Autodesk Inventor part; units mm, degrees
ref_plane "YZ Plane" through (0, 0, 0) normal (1, 0, 0) x (0, 1, 0)
ref_plane "XZ Plane" through (0, 0, 0) normal (0, 1, 0) x (-1, 0, 0)
ref_plane "XY Plane" through (0, 0, 0) normal (0, 0, 1) x (1, 0, 0)
sketch "スケッチ1" plane through (0, 0, 0) normal (0, 1, 0) x (-1, 0, 0)
  circle A0 centre (0, 0) radius 178.1675
  circle A1 centre (0, 0) radius 157.8276
  line L0 (168.1877, 0) -> (166.7488, -21.9529)
  line L1 (168.1877, 0) -> (130.1721, 2.4917) construction
  line L2 (249.4344, 0) -> (-249.4344, 0)
  line L3 (166.7488, -21.9529) -> (156.7702, -21.2989)
  line L4 (156.7702, -21.2989) -> (158.2091, 0.654) construction
  line L5 (158.2091, 0.654) -> (168.1877, 0)
  line L6 (157.4896, -10.3224) -> (0, 0)
  line L7 (166.7488, -21.9529) -> (162.4568, -43.5302)
  line L8 (162.4568, -43.5302) -> (152.649, -41.5793) construction
  line L9 (152.649, -41.5793) -> (156.9409, -20.002) construction
  line L10 (156.9409, -20.002) -> (166.7488, -21.9529) construction
  line L11 (162.4568, -43.5302) -> (155.3851, -64.3626)
  line L12 (155.3851, -64.3626) -> (145.9158, -61.1482) construction
  line L13 (145.9158, -61.1482) -> (152.9875, -40.3158) construction
  line L14 (152.9875, -40.3158) -> (162.4568, -43.5302) construction
  line L15 (155.3851, -64.3626) -> (145.6548, -84.0938)
  line L16 (145.6548, -84.0938) -> (136.6861, -79.6709) construction
  line L17 (136.6861, -79.6709) -> (146.4164, -59.9397) construction
  line L18 (146.4164, -59.9397) -> (155.3851, -64.3626) construction
  line L19 (0, 0) -> (111.6009, -111.6009)
  line L20 (145.6548, -84.0938) -> (137.3401, -78.5381) construction
  line L21 (137.3401, -78.5381) -> (125.1176, -96.8305) construction
  line L22 (125.1176, -96.8305) -> (133.4323, -102.3862) construction
  line L23 (133.4323, -102.3862) -> (145.6548, -84.0938)
  line L24 (133.4323, -102.3862) -> (125.9139, -95.7927) construction
  line L25 (125.9139, -95.7927) -> (111.4082, -112.3332) construction
  line L26 (111.4082, -112.3332) -> (118.9266, -118.9266)
  line L27 (118.9266, -118.9266) -> (133.4323, -102.3862)
  line L28 (111.6009, -111.6009) -> (118.9266, -118.9266)
  line L29 (166.7488, -21.9529) -> (176.7274, -22.6069) construction
  line L30 (118.9266, -118.9266) -> (125.9834, -125.9834)
  point P0 (154.795, -30.7906)
  point P1 (149.4517, -50.732)
  point P2 (141.5512, -69.8053)
  point P3 (131.2288, -87.6843)
  point P4 (118.661, -104.0629)
  point P5 (157.8276, 0)
  point P6 (178.1675, 0)
  dimension "d0" = 22
  dimension "d1" = 10
  dimension "d2" = 45
  dimension "d4" = 315.6551
extrude "押し出し1" add sketch "スケッチ1" along normal blind 5.5 contours L30 L27 L23 L15 L11 L7 L0 L2 A0 | L28 A1 L2 L0 L7 L11 L15 L23 L27
sketch "スケッチ2" plane through (0, 5.5, 0) normal (0, 1, 0) x (1, 0, 0)
  circle A0 centre (0, 0) radius 277.8276
  line L0 (-168.1877, 0) -> (-166.7488, 21.9529)
  line L1 (-166.7488, 21.9529) -> (-162.4568, 43.5302)
  line L2 (-162.4568, 43.5302) -> (-155.3851, 64.3626)
  line L3 (-155.3851, 64.3626) -> (-145.6548, 84.0938)
  line L4 (-133.4323, 102.3862) -> (-145.6548, 84.0938)
  line L5 (-118.9266, 118.9266) -> (-133.4323, 102.3862)
  line L6 (-167.4682, 10.9764) -> (-166.0294, 32.9293)
  line L7 (-166.0294, 32.9293) -> (-275.7938, 40.1237)
  line L8 (-275.7938, 40.1237) -> (-277.2327, 18.1708)
  line L9 (-277.2327, 18.1708) -> (-167.4682, 10.9764)
  line L10 (-164.6028, 32.7415) -> (-160.3108, 54.3188)
  line L11 (-160.3108, 54.3188) -> (-268.1972, 75.7787)
  line L12 (-268.1972, 75.7787) -> (-272.4892, 54.2015)
  line L13 (-272.4892, 54.2015) -> (-164.6028, 32.7415)
  circle A1 centre (-166.7488, 21.9529) radius 11
  circle A2 centre (-162.4568, 43.5302) radius 11
  line L14 (-158.921, 53.9464) -> (-151.8493, 74.7789)
  line L15 (-151.8493, 74.7789) -> (-256.0116, 110.1372)
  line L16 (-256.0116, 110.1372) -> (-263.0833, 89.3047)
  line L17 (-263.0833, 89.3047) -> (-158.921, 53.9464)
  circle A3 centre (-155.3851, 64.3626) radius 11
  arc A4 (-275.7591, 62.4834) -> (-281.3553, 41.7349) centre (-166.7488, 21.9529) ccw
  line L18 (-178.1663, 0.654) -> (-158.2091, -0.654)
  line L19 (-158.2091, -0.654) -> (-156.7702, 21.2989)
  line L20 (-156.7702, 21.2989) -> (-176.7274, 22.6069)
  line L21 (-176.7274, 22.6069) -> (-178.1663, 0.654)
  line L22 (-177.4468, 11.6305) -> (-275.7938, 40.1237)
  line L23 (-176.7274, 22.6069) -> (-176.008, 33.5834)
  line L24 (-176.008, 33.5834) -> (-275.7591, 62.4834)
  line L25 (-275.7938, 40.1237) -> (-281.3553, 41.7349)
  circle A5 centre (0, 0) radius 137.8276
  line L26 (0, 0) -> (-196.4538, 196.4538)
  line L27 (-111.6009, 111.6009) -> (-125.9834, 125.9834)
  line L28 (-433.7586, 0) -> (433.7586, 0)
  circle A6 centre (0, 0) radius 257.8276 construction
  arc A7 (-111.6009, 111.6009) -> (-157.8276, 0) centre (0, 0) ccw
  point P0 (-158.1662, 0)
  point P1 (-137.8276, 0)
  point P2 (-97.4588, 97.4588)
  point P3 (-277.8276, 0)
  dimension "d7" = 22
  dimension "d10" = 20
  dimension "d11" = 100
  dimension "d12" = 20
  dimension "d14" = 20
  dimension "d17" = 100
extrude "押し出し2" add sketch "スケッチ2" against normal blind 5.5 contours L26 L5 L4 L3 A3 L15 A0 | A0 L9 L21 L18 L28 | L15 A3 L17 A0 | A0 L22 L9 | L18 L21 L9 L0 | L0 A1 L19 L28 | A5 L28 A7 A1 A2 A3 L26 | L17 A2 L11 A0 | A3 L3 L14 | L14 L2 A3 | L26 A7 A3 L3 L4 L5 | A0 L7 L23 A1 L21 L22 | L21 A1 L9 | A1 L21 L20 L0 | L0 L20 L19 A1 | L19 A7 L28 | L11 A2 L13 L24 A0 | A2 A7 L1 L2 | L2 L10 A2 | A3 A7 A2 | L2 L3 A3 A7 | A0 L13 L24 L7 | A1 L23 L21 | L6 A1 L1 | L20 L23 A1 L6 | L1 A1 A7 L19 L20 | A1 A7 L19 | A3 A7 | L24 L13 A0 | L10 L1 A2 | A2 A7 | L24 L13 A1 L7 | L7 A1 L23 | A2 A7 A1 | A7 A1
sketch "スケッチ3" plane through (0, 5.5, 0) normal (0, 1, 0) x (1, 0, 0)
  circle A0 centre (0, 0) radius 257.8276
  arc A1 (-97.4588, 97.4588) -> (-137.8276, 0) centre (0, 0) ccw
  line L0 (-97.4588, 97.4588) -> (-196.4538, 196.4538)
  line L1 (-277.8276, 0) -> (-137.8276, 0)
  arc A2 (-196.4538, 196.4538) -> (-277.8276, 0) centre (0, 0) ccw
  point P0 (-257.8276, 0)
  point P1 (-182.3116, 182.3116)
  dimension "d21" = 20
extrude "押し出し3" cut sketch "スケッチ3" against normal through all contours L0 A1 L1 A0 picked at (-202.0143, 80.8888)
sketch "スケッチ5" plane through (0, 5.5, 0) normal (0, 1, 0) x (1, 0, 0)
  line L0 (-196.4538, 196.4538) -> (-182.3116, 182.3116)
  line L1 (-196.4538, 196.4538) -> (-189.3827, 203.5248)
  line L2 (-189.3827, 203.5248) -> (-181.6045, 195.7467)
  line L3 (-181.6045, 195.7467) -> (-190.0898, 190.0898)
  line L4 (-189.3827, 189.3827) -> (-192.1791, 186.5862)
  line L5 (-182.3116, 182.3116) -> (-196.4538, 196.4538)
  point P0 (0, 0)
  dimension "d30" = 1
  dimension "d31" = 1
  dimension "d33" = 10
extrude "押し出し5" add sketch "スケッチ5" against normal up to surface (5.5 mm away)
sketch "スケッチ6" plane through (0, 5.5, 0) normal (0, 1, 0) x (1, 0, 0)
  line L0 (-277.8276, 0) -> (-277.8276, 10.5)
  line L1 (-277.8276, 10.5) -> (-266.3276, 10.5)
  line L2 (-266.3276, 10.5) -> (-268.3276, 0)
  line L3 (-257.8276, 0) -> (-277.8276, 0)
  line L4 (-277.8276, 0) -> (-257.8276, 0)
  point P0 (0, 0)
  point P1 (-267.8276, 0)
  point P2 (-267.8276, 0)
  dimension "d36" = 0.5
  dimension "d37" = 1.5
  dimension "d38" = 10.5
extrude "押し出し6" cut sketch "スケッチ6" against normal through all
sketch "スケッチ7" plane through (0, 5.5, 0) normal (0, 1, 0) x (1, 0, 0)
  line L0 (0, 0) -> (-254.6239, 111.1523) construction
  line L1 (-182.3116, 182.3116) -> (-190.0898, 190.0898)
  line L2 (0, 0) -> (-182.3116, 182.3116) construction
  line L3 (-277.6291, 10.5) -> (-266.3276, 10.5)
  line L4 (0, 0) -> (-277.6291, 10.5) construction
  arc A0 (-196.4538, 196.4538) -> (-277.6291, 10.5) centre (0, 0) ccw
  line L5 (-256.6243, 106.5698) -> (-252.6235, 115.7347) construction
  line L6 (-252.6235, 115.7347) -> (-249.8741, 114.5344)
  line L7 (-249.8741, 114.5344) -> (-253.8748, 105.3696)
  line L8 (-253.8748, 105.3696) -> (-256.6243, 106.5698)
  line L9 (-238.2947, 98.5683) -> (-234.2939, 107.7331) construction
  line L10 (-234.2939, 107.7331) -> (-237.0433, 108.9334)
  line L11 (-237.0433, 108.9334) -> (-241.0441, 99.7685)
  line L12 (-241.0441, 99.7685) -> (-238.2947, 98.5683)
  arc A1 (-182.3116, 182.3116) -> (-257.8276, 0) centre (0, 0) ccw
  line L13 (-238.2947, 98.5683) -> (-238.2502, 98.5489)
  arc A2 (-182.3116, 182.3116) -> (-257.8276, 0) centre (0, 0) ccw
  line L14 (-234.2939, 107.7331) -> (-234.2495, 107.7137)
  point P0 (-236.2943, 103.1507)
  point P1 (-252.5823, 115.7167)
  point P2 (-256.5831, 106.5518)
  dimension "d41" = 3
  dimension "d42" = 10
extrude "押し出し7" cut sketch "スケッチ7" against normal through all
pattern_circular "円形状パターン1" count 2 over 15 about axis through (0, -10, 0) along (0, 1, 0) of "押し出し7"
pattern_circular "円形状パターン2" count 2 over 15 about axis through (0, -10, 0) along (0, -1, 0) of "押し出し7"
properties part number "front_under" material "木材 (カエデ材)"
For this review, take the finished solid that the model builds, in its own axes (mm). A direction names the side the tool comes from. Give positions to 0.01 mm unless a question says otherwise; leave off trailing zeros. Loops run counter-clockwise (first coordinate to the right, second up) from the corner with the lowest first, then second, coordinate; pieces in that order, holes last. Notation, with made-up numbers: M 51.5,71 L 82.5,71 A6 ccw 82.5,76 Z; hole C 43.25,80 d1. An arc over 180 degrees is marked long. One line per item, written item: value. Start each with the question number.
Q1. For L1, parallel to X at y = 1.7, z = -108.5; L2, parallel to X at y = 0.95, z = -41; L3, parallel to Z at x = -234.5, y = 1.3, list the stretches that pass through material, from the lowest coordinate up.
Q2. Add section B-B (x = -223.5). Give the boundary of the cut face in (y, z), and give its area (3 significant figures).
Q3. Add section A-A (z = -154.5). Give the boundary of the cut face in (x, y).
Q4. Draft analysis for pull direction X (two halves, no side actions). For faces 1 (the face through (-237.71, 2.79, -143.81)), 2 (the face through (-263, 3, 0)), 3 (the face through (-214.79, 2.79, -171.45)), 4 (the face through (-203.847, 2.788, -162.719)), state which applies: released by +X, released by -X, zero draft, split by the parting line, or undercut.
Q5. Machinability: for faces 5 (the face through (-185.788, 2.788, -192.958)), 6 (the face through (-185.55, 2.79, -199.69)), 7 (the face through (-272, 3, -10.5)), which of the approach directions +Z, -Z, +X, -X, +Y, -Y give a long, thin tool a straight path to every point of the face, cutting with its end or side? Answer none if there is none.
Reply:
1. L1: -252.51 to -237.23, -236.05 to -233.89
1. L2: -271.75 to -257.59
1. L3: -148.99 to -107.82
2. outline: M 0,-165.03 L 5.5,-165.03 L 5.5,-128.54 L 0,-128.54 Z
2. area: 201 mm²
3. outline: M -230.91,0 L -206.41,0 L -206.41,5.5 L -230.91,5.5 Z
4. face 1: released by -X
4. face 2: zero draft
4. face 3: undercut
4. face 4: undercut
5. face 5: +X, +Y, -Y
5. face 6: -Z, +X, +Y, -Y
5. face 7: -X, +Y, -Y
